For this review, take the finished solid that the model builds, in its own axes (mm). Give positions to 0.01 mm unless a question says otherwise; leave off trailing zeros. Write each loop counter-clockwise with the first axis right and the second up, starting at its lowest first coordinate (ties: lowest second). Pieces come first, ordered by that corner, then holes. Notation, with made-up numbers: M 58,-8.75 L 116,-8.75 A16 cw 116,3.25 Z; hole C 12,-7 d7. An arc over 180 degrees is marked long. One line per item, written item: value. Start each with the question number.
Item 1: Consider section B-B, the plane x = 202.5. Write out the cut boundary in (y, z).
Item 2: Consider section A-A, the plane y = 2.75. Write out the cut boundary in (x, z).
Item 3: Clearance check with flat-ended pins moving along their axes: pin 1 Ø2.5 at (y, z) = (7.5, 56.5) entering from -X; pin 2 Ø2.5 at (x, z) = (380.8, 31.5) entering from -Y; pin 3 Ø1.5 at (y, z) = (7.5, 57) entering from +X. State where each tip first meets the part, or that it passes through.
Item 4: To check wall thickness, follow probe 1 along X at (y, z) = (11.75, 56.5); probe 2 along Y at (x, z) = (389.5, 31.5); probe 3 along Z at (x, y) = (181, 5.75). State the ranges of each line that lie inside material, in increasing order.
```python
from build123d import *

# Parameters (mm, degrees)
SKETCH_W        = 395.8
SKETCH_H        = 64
PAD_DEPTH       = 15
SKETCH001_R     = 1.5
POCKET_DEPTH    = 15.001
SKETCH002_W     = 395.8
SKETCH002_H     = 4
POCKET001_DEPTH = 7.5
SKETCH003_R     = 1.5
POCKET002_DEPTH = 20
SKETCH004_R     = 1.5
POCKET003_DEPTH = 20
POCKET004_DEPTH = 15.001


with BuildPart() as part:
    # Sketch → Pad (new body)
    with BuildSketch(Plane.XZ):
        with Locations((197.9, 32)):
            Rectangle(SKETCH_W, SKETCH_H)
    extrude(amount=-PAD_DEPTH)

    # Sketch001 (on Face5 of Pad) → Pocket (cut, through all)
    with BuildSketch(Plane.XZ):
        with Locations((15, 56.5)):
            Circle(SKETCH001_R)
        with Locations((15, 31.5)):
            Circle(SKETCH001_R)
        with Locations((380.8, 31.5)):
            Circle(SKETCH001_R)
        with Locations((380.8, 56.5)):
            Circle(SKETCH001_R)
        with Locations((15, 10)):
            Circle(SKETCH001_R)
        with Locations((380.8, 10)):
            Circle(SKETCH001_R)
    extrude(amount=-POCKET_DEPTH, mode=Mode.SUBTRACT)

    # Sketch002 (on Face4 of Pocket) → Pocket001 (cut)
    with BuildSketch(Plane.XZ):
        with Locations((197.9, 22)):
            Rectangle(SKETCH002_W, SKETCH002_H)
    extrude(amount=-POCKET001_DEPTH, mode=Mode.SUBTRACT)

    # Sketch003 (on Face3 of Pocket001) → Pocket002 (cut)
    with BuildSketch(Plane(origin=(395.8, 0, 0), x_dir=(0, 0, 1), z_dir=(1, 0, 0))):
        with Locations((10, -7.5)):
            Circle(SKETCH003_R)
        with Locations((31.5, -7.5)):
            Circle(SKETCH003_R)
        with Locations((56.5, -7.5)):
            Circle(SKETCH003_R)
    extrude(amount=-POCKET002_DEPTH, mode=Mode.SUBTRACT)

    # Sketch004 (on Face2 of Pocket002) → Pocket003 (cut)
    with BuildSketch(Plane(origin=(0, 0, 0), x_dir=(0, 0, -1), z_dir=(-1, 0, 0))):
        with Locations((-56.5, -7.5)):
            Circle(SKETCH004_R)
        with Locations((-31.5, -7.5)):
            Circle(SKETCH004_R)
        with Locations((-10, -7.5)):
            Circle(SKETCH004_R)
    extrude(amount=-POCKET003_DEPTH, mode=Mode.SUBTRACT)

    # Sketch005 (on Face5 of Pocket003) → Pocket004 (cut, through all)
    with BuildSketch(Plane(origin=(0, 15, 0), x_dir=(1, 0, 0), z_dir=(0, 1, 0))):
        with BuildLine():
            Line((0, -51.5), (13, -51.5))
            ThreePointArc((13, -51.5), (14.414214, -50.914214), (15, -49.5))
            Line((15, -49.5), (15, -38.5))
            ThreePointArc((15, -38.5), (14.414214, -37.085786), (13, -36.5))
            Line((13, -36.5), (0, -36.5))
            Line((0, -36.5), (0, -51.5))
        make_face()
        with BuildLine():
            Line((395.8, -51.5), (382.8, -51.5))
            ThreePointArc((380.8, -49.5), (381.385786, -50.914214), (382.8, -51.5))
            Line((380.8, -49.5), (380.8, -38.5))
            ThreePointArc((382.8, -36.5), (381.385786, -37.085786), (380.8, -38.5))
            Line((382.8, -36.5), (395.8, -36.5))
            Line((395.8, -36.5), (395.8, -44))
            Line((395.8, -44), (395.8, -51.5))
        make_face()
    extrude(amount=-POCKET004_DEPTH, mode=Mode.SUBTRACT)


solid = part.part
```
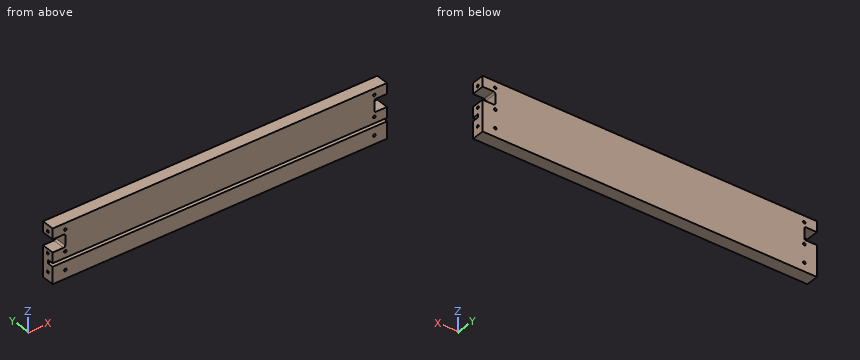
Model answer:
1. outline: M 0,0 L 15,0 L 15,64 L 0,64 L 0,24 L 7.5,24 L 7.5,20 L 0,20 Z
2. outline: M 0,0 L 395.8,0 L 395.8,20 L 0,20 Z; M 0,24 L 395.8,24 L 395.8,36.5 L 382.8,36.5 A2 cw 380.8,38.5 L 380.8,49.5 A2 cw 382.8,51.5 L 395.8,51.5 L 395.8,64 L 0,64 L 0,51.5 L 13,51.5 A2 cw 15,49.5 L 15,38.5 A2 cw 13,36.5 L 0,36.5 Z; hole C 15,10 d3; hole C 15,31.5 d3; hole C 15,56.5 d3; hole C 380.8,10 d3; hole C 380.8,31.5 d3; hole C 380.8,56.5 d3
3. pin 1: stops at x = 20
3. pin 2: passes through
3. pin 3: stops at x = 375.8
4. probe 1: x = 0 to 13.5, 16.5 to 379.3, 382.3 to 395.8
4. probe 2: y = 0 to 6, 9 to 15
4. probe 3: z = 0 to 20, 24 to 64
